Geometry check sheet. Reference: the model listing, model coordinates, mm. Face numbers are marked on the shaded views. A direction names the side the tool comes from. Give positions to 0.01 mm unless a question says otherwise; leave off trailing zeros. Write each loop counter-clockwise with the first axis right and the second up, starting at its lowest first coordinate (ties: lowest second). Pieces come first, ordered by that corner, then holes. Notation, with made-up numbers: M 63.5,-23.75 L 80.5,-23.75 A17 ccw 80.5,-17.75 Z; hole C 25.5,-7 d9. An arc over 180 degrees is marked long. One line per item, written item: value. Start each with the question number.
1. Gauge pin test, flat ends, axial feed: pin 1 (2 mm diameter, centred on y = -117, z = 82.5, fed in from +X); pin 2 (1.7 mm diameter, centred on y = 53.5, z = 10, fed in from +X); pin 3 (2 mm diameter, centred on x = 39.5, y = -19, fed in from +Z). Record the tip position at first contact, or that the pin passes through.
2. Cross-section at A-A on y = -98.5. Record the cut outline in (x, z).
3. Tool access check on the marked faces 4 and 5. Record the directions out of +Z, -Z, +X, -X, +Y, -Y that give a thin tool (end or side, any length) a straight path to the whole face; none if there is none.
4. Cross-section at D-D on z = 43. Record the cut outline in (x, y).
5. Scan lines: line 1 (Z direction, x = 24.5, y = -80.5); line 2 (Y direction, x = -34.5, z = 27.5); line 3 (X direction, y = -5.5, z = 5). Record each from-to range of solid material in increasing order.
6. Cross-section at C-C on y = 16. Record the cut outline in (x, z).
7. Release check for a two-part mould opening along Z. For the marked faces 1, 2 and 3 record: pulls with the +Z half, pulls with the -Z half, needs draft (parallel to the pull), parting line crosses it, or undercut.
8. Cross-section at B-B on x = -1. Record the cut outline in (y, z), then the cut area to 3 significant figures.
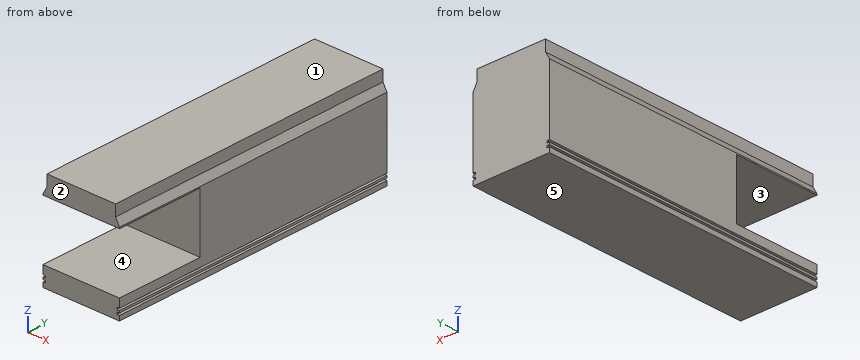
from build123d import *

# Parameters (mm, degrees)
F0_W     = 80
F0_H     = 300
F1_DEPTH = 100
F3_W     = 90.5103512108
F3_H     = 60.133138299
F4_DEPTH = 128
F2_W     = 2.603494525
F2_H     = 2.1046474576
F5_DEPTH = 322.9


with BuildPart() as f1:
    # F0 (on Top) → F1 (new body)
    with BuildSketch(Plane.XY):
        Rectangle(F0_W, F0_H)
    extrude(amount=F1_DEPTH)

    # F3 (on face) → F4 (cut)
    with BuildSketch(Plane.YZ.offset(40)):
        with Locations((-104.7448243946, 50)):
            Rectangle(F3_W, F3_H)
    extrude(amount=-F4_DEPTH, mode=Mode.SUBTRACT)

    # F2 (on face) → F5 (cut)
    with BuildSketch(Plane.XZ.offset(150)):
        Polygon((40, 100), (35.7759818435, 100), (35.7759818435, 88.739156723), (40, 81.3345983624), align=None)
        Polygon((-35.7759818435, 88.739156723), (-35.7759818435, 100), (-40, 100), (-40, 81.3345983624), align=None)
        with Locations((38.6982527375, 10.1477000862)):
            Rectangle(F2_W, F2_H)
        with Locations((38.6982527375, 5.938405171)):
            Rectangle(F2_W, F2_H)
        with Locations((-38.6982527375, 5.938405171)):
            Rectangle(F2_W, F2_H)
        with Locations((-38.6982527375, 10.1477000862)):
            Rectangle(F2_W, F2_H)
    extrude(amount=-F5_DEPTH, mode=Mode.SUBTRACT)


solid = f1.part
Report:
1. pin 1: stops at x = 39.91
1. pin 2: stops at x = 37.4
1. pin 3: stops at z = 83.96
2. outline: M -40,0 L 40,0 L 40,4.89 L 37.4,4.89 L 37.4,6.99 L 40,6.99 L 40,9.1 L 37.4,9.1 L 37.4,11.2 L 40,11.2 L 40,19.93 L -40,19.93 L -40,11.2 L -37.4,11.2 L -37.4,9.1 L -40,9.1 L -40,6.99 L -37.4,6.99 L -37.4,4.89 L -40,4.89 Z; M -40,80.07 L 40,80.07 L 40,81.33 L 35.78,88.74 L 35.78,100 L -35.78,100 L -35.78,88.74 L -40,81.33 Z
3. face 4: +X, -X, -Y
3. face 5: -Z, +X, -X, +Y, -Y
4. outline: M -40,-59.49 L 40,-59.49 L 40,150 L -40,150 Z
5. line 1: z = 0 to 19.93, 80.07 to 100
5. line 2: y = -59.49 to 150
5. line 3: x = -37.4 to 37.4
6. outline: M -40,0 L 40,0 L 40,4.89 L 37.4,4.89 L 37.4,6.99 L 40,6.99 L 40,9.1 L 37.4,9.1 L 37.4,11.2 L 40,11.2 L 40,81.33 L 35.78,88.74 L 35.78,100 L -35.78,100 L -35.78,88.74 L -40,81.33 L -40,11.2 L -37.4,11.2 L -37.4,9.1 L -40,9.1 L -40,6.99 L -37.4,6.99 L -37.4,4.89 L -40,4.89 Z
7. face 1: pulls with the +Z half
7. face 2: needs draft
7. face 3: undercut
8. outline: M -150,0 L 150,0 L 150,100 L -150,100 L -150,80.07 L -59.49,80.07 L -59.49,19.93 L -150,19.93 Z
8. area: 24,600 mm^2
